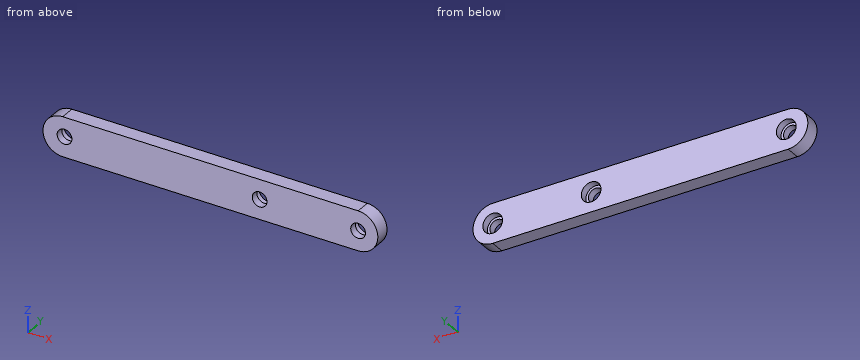
from build123d import *

# Parameters (mm, degrees)
SKETCH1_R           = 3
BOSS_EXTRUDE1_DEPTH = 6
SKETCH3_R           = 4
CUT_EXTRUDE1_DEPTH  = 3


with BuildPart() as part:
    # Sketch1 → Boss-Extrude1 (new body)
    with BuildSketch(Plane(origin=(0, 0, 0), x_dir=(1, 0, 0), z_dir=(0, 1, 0))):
        with BuildLine():
            Line((-60, -8), (60, -8))
            ThreePointArc((60, -8), (68, 0), (60, 8))
            Line((60, 8), (-60, 8))
            ThreePointArc((-60, 8), (-68, 0), (-60, -8))
        make_face()
        with Locations(Location((-59.243309237, -0.211557176, 0), (0, 0, 270))):
            Circle(SKETCH1_R, mode=Mode.SUBTRACT)
        with Locations(Location((60, 0, 0), (0, 0, 270))):
            Circle(SKETCH1_R, mode=Mode.SUBTRACT)
        with Locations(Location((20, 0, 0), (0, 0, 270))):
            Circle(SKETCH1_R, mode=Mode.SUBTRACT)
    extrude(amount=BOSS_EXTRUDE1_DEPTH)

    # Sketch3 → Cut-Extrude1 (cut)
    with BuildSketch(Plane(origin=(0, 6, 0), x_dir=(1, 0, 0), z_dir=(0, 1, 0))):
        with Locations(Location((-59.243309237, -0.211557176, 0), (0, 0, 270))):
            Circle(SKETCH3_R)
        with Locations(Location((20, 0, 0), (0, 0, 270))):
            Circle(SKETCH3_R)
        with Locations(Location((60, 0, 0), (0, 0, 270))):
            Circle(SKETCH3_R)
    extrude(amount=-CUT_EXTRUDE1_DEPTH, mode=Mode.SUBTRACT)


solid = part.part
Design review of the part built by this model. Coordinates are the model's own, in mm. Round coordinates to 2 decimals unless told otherwise and drop trailing zeros. Order: outer loops, then holes, each group sorted by start corner. A loop starts at its lowest first (then second) coordinate and runs counter-clockwise, first axis right, second up. Notation, with made-up numbers: M 41,37.25 L 53,37.25 A12 ccw 53,48.25 Z; hole C 71.5,-2 d6. An arc over 180 degrees is marked long. Answer as CSV lines item,"result". Start each with the question number.
1) Add section C-C (y = 4.05). Give the boundary of the cut face in (x, z).
2) Wall thickness on line 1 along X through (y, z) = (5.4, 0.25); line 2 along X through (y, z) = (0.85, 0); line 3 along Z through (x, y) = (-59, 5.6): over which ranges is each line inside the solid? List them lowest first. Write a range as [from, to].
3) For pin 1 Ø5 at (x, z) = (-59.24, 0.21) entering from -Y; pin 2 Ø2.5 at (x, z) = (-61, 1.5) entering from +Y, all flat-tipped, find the tip position at first contact; note any pin that passes through.
4) Add section B-B (z = 1.75). Give the boundary of the cut face in (x, y), then the cut area to 3 significant figures.
5) Add section A-A (x = 20). Give the boundary of the cut face in (y, z).
6) Add section D-D (z = -5.5). Give the boundary of the cut face in (x, y).
Resolved:
1,outline,"M -60,-8 L 60,-8 A8 ccw 60,8 L -60,8 A8 ccw Z; hole C -59.24,0.21 d8; hole C 20,0 d8; hole C 60,0 d8"
2,line 1,"[-68, -63.24], [-55.24, 16.01], [23.99, 56.01], [63.99, 68]"
2,line 2,"[-68, -62.24], [-56.25, 17], [23, 57], [63, 68]"
2,line 3,"[-8, -3.78], [4.2, 8]"
3,pin 1,"through"
3,pin 2,"y = 3"
4,outline,"M -67.81,0 L -61.82,0 L -61.82,3 L -62.94,3 L -62.94,6 L -67.81,6 Z; M -56.67,0 L 17.56,0 L 17.56,3 L 16.4,3 L 16.4,6 L -55.55,6 L -55.55,3 L -56.67,3 Z; M 22.44,0 L 57.56,0 L 57.56,3 L 56.4,3 L 56.4,6 L 23.6,6 L 23.6,3 L 22.44,3 Z; M 62.44,0 L 67.81,0 L 67.81,6 L 63.6,6 L 63.6,3 L 62.44,3 Z"
4,area,"704 mm^2"
5,outline,"M 0,-8 L 6,-8 L 6,-4 L 3,-4 L 3,-3 L 0,-3 Z; M 0,3 L 3,3 L 3,4 L 6,4 L 6,8 L 0,8 Z"
6,outline,"M -65.81,0 L 65.81,0 L 65.81,6 L -65.81,6 Z"
